Verification items for the finished model (mm, model axes). Face numbers are marked on the shaded views. A direction names the side the tool comes from. Give positions to 0.01 mm unless a question says otherwise; leave off trailing zeros. Loops run counter-clockwise (first coordinate to the right, second up) from the corner with the lowest first, then second, coordinate; pieces in that order, holes last. Notation, with made-up numbers: (35, 16) - (79, 16) arc R27 ccw to (79, 46) - close; hole circle Ø4 at (73.25, -9). An arc over 180 degrees is marked (long way). One line per item, written item: value. Start each with the question number.
1. Mould release check, pull along X, two halves, no side actions. Record for the marked faces 5 and 6: pulls with the +X half, pulls with the -X half, needs draft (parallel to the pull), parting line crosses it, or undercut.
2. Sectioned sample at C-C (z = 2.4). Count the separate pieces of the cut face and the enclosed holes in it, plus the area to 3 significant figures.
3. Access from +Z, -Z, +X, -X, +Y, -Y to the whole of each face (thin tool, end or side, straight path). Record for the marked faces 1, 2, 3 and 4.
4. Sectioned sample at D-D (x = 10). Record the cut outline in (y, z), plus the area to 3 significant figures.
5. Sectioned sample at B-B (y = 0). Record the cut outline in (x, z).
6. Gauge pin test, flat ends, axial feed: pin 1 (1.2 mm diameter, centred on y = 21, z = 2.5, fed in from +X); pin 2 (1.2 mm diameter, centred on x = 0.5, z = 2, fed in from -Y); pin 3 (3 mm diameter, centred on y = -2.5, z = 2, fed in from -X). Record the tip position at first contact, or that the pin passes through.
7. Sectioned sample at A-A (x = -1). Record the cut outline in (y, z).
8. Scan lines: L1, parallel to Y at x = 3, z = 2.85; L2, parallel to X at y = 21, z = 2.4; L3, parallel to X at y = 10, z = 3.75. Record each from-to range of solid material in increasing order. Write a range as [from, to].
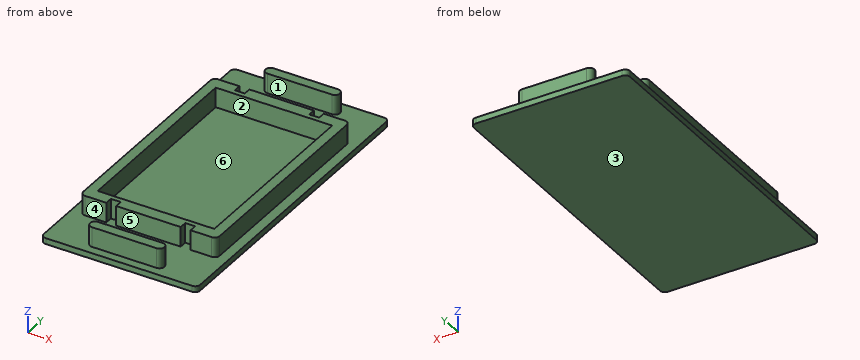
from build123d import *

# Parameters (mm, degrees)
F0_W     = 31.5
F0_H     = 63.5
F0_W_2   = 23.5
F0_H_2   = 39
F0_W_3   = 15
F0_H_3   = 2
F0_W_4   = 2
F0_H_4   = 1.5
F1_DEPTH = 1.2
F2_DEPTH = 4
F3_R     = 0.99999


# Not quite as in the source:
# - a fillet or chamfer is up to 0.001 mm smaller than in the source, because OpenCascade refuses the exact size


with BuildPart() as f1:
    # F0 (on Top) → F1 (new body)
    with BuildSketch(Plane.XY):
        Rectangle(F0_W, F0_H)
        Polygon((13.75, -22), (13.75, -30), (7.5, -30), (-7.5, -30), (-13.75, -30), (-13.75, -22), (-13.75, 22), (-13.75, 30), (-7.5, 30), (7.5, 30), (13.75, 30), (13.75, 22), align=None, mode=Mode.SUBTRACT)
        Rectangle(F0_W_2, F0_H_2)
        Polygon((-7.5, -28), (7.5, -28), (11.75, -28), (11.75, -22), (8.5, -22), (6.5, -22), (-6.5, -22), (-8.5, -22), (-11.75, -22), (-11.75, -28), align=None)
        Polygon((8.5, 22), (11.75, 22), (11.75, 28), (7.5, 28), (-7.5, 28), (-11.75, 28), (-11.75, 22), (-8.5, 22), (-6.5, 22), (6.5, 22), align=None)
        Polygon((-13.75, 22), (-13.75, -22), (-11.75, -22), (-11.75, -19.5), (-11.75, 19.5), (-11.75, 22), align=None)
        Polygon((11.75, -22), (13.75, -22), (13.75, 22), (11.75, 22), (11.75, 19.5), (11.75, -19.5), align=None)
        Polygon((8.5, -22), (11.75, -22), (11.75, -19.5), (-11.75, -19.5), (-11.75, -22), (-8.5, -22), (-8.5, -20.5), (-6.5, -20.5), (-6.5, -22), (6.5, -22), (6.5, -20.5), (8.5, -20.5), align=None)
        Polygon((11.75, 19.5), (11.75, 22), (8.5, 22), (8.5, 20.5), (6.5, 20.5), (6.5, 22), (-6.5, 22), (-6.5, 20.5), (-8.5, 20.5), (-8.5, 22), (-11.75, 22), (-11.75, 19.5), align=None)
        with Locations((0, -29)):
            Rectangle(F0_W_3, F0_H_3)
        with Locations((0, 29)):
            Rectangle(F0_W_3, F0_H_3)
        Polygon((7.5, -30), (13.75, -30), (13.75, -22), (11.75, -22), (11.75, -28), (7.5, -28), align=None)
        Polygon((-13.75, -30), (-7.5, -30), (-7.5, -28), (-11.75, -28), (-11.75, -22), (-13.75, -22), align=None)
        Polygon((11.75, 22), (13.75, 22), (13.75, 30), (7.5, 30), (7.5, 28), (11.75, 28), align=None)
        Polygon((-13.75, 30), (-13.75, 22), (-11.75, 22), (-11.75, 28), (-7.5, 28), (-7.5, 30), align=None)
        with Locations((-7.5, 21.25)):
            Rectangle(F0_W_4, F0_H_4)
        with Locations((7.5, 21.25)):
            Rectangle(F0_W_4, F0_H_4)
        with Locations((-7.5, -21.25)):
            Rectangle(F0_W_4, F0_H_4)
        with Locations((7.5, -21.25)):
            Rectangle(F0_W_4, F0_H_4)
    extrude(amount=-F1_DEPTH)

    # F0 (on Top) → F2 (join)
    with BuildSketch(Plane.XY):
        Polygon((-13.75, 22), (-13.75, -22), (-11.75, -22), (-11.75, -19.5), (-11.75, 19.5), (-11.75, 22), align=None)
        Polygon((11.75, 19.5), (11.75, 22), (8.5, 22), (8.5, 20.5), (6.5, 20.5), (6.5, 22), (-6.5, 22), (-6.5, 20.5), (-8.5, 20.5), (-8.5, 22), (-11.75, 22), (-11.75, 19.5), align=None)
        Polygon((11.75, -22), (13.75, -22), (13.75, 22), (11.75, 22), (11.75, 19.5), (11.75, -19.5), align=None)
        Polygon((8.5, -22), (11.75, -22), (11.75, -19.5), (-11.75, -19.5), (-11.75, -22), (-8.5, -22), (-8.5, -20.5), (-6.5, -20.5), (-6.5, -22), (6.5, -22), (6.5, -20.5), (8.5, -20.5), align=None)
        with Locations((0, 29)):
            Rectangle(F0_W_3, F0_H_3)
        with Locations((0, -29)):
            Rectangle(F0_W_3, F0_H_3)
    extrude(amount=F2_DEPTH)

    # F3 (radius 1 in the source; OpenCascade refuses exactly that, so slightly less here)
    f3_edges = [f1.edges().sort_by_distance(p)[0] for p in [
        (-13.75, 22, 2),
        (13.75, 22, 2),
        (13.75, -22, 2),
        (-13.75, -22, 2),
        (-15.75, -31.75, -0.6),
        (15.75, -31.75, -0.6),
        (-15.75, 31.75, -0.6),
        (15.75, 31.75, -0.6),
        (-7.5, -30, 2),
        (7.5, -30, 2),
        (7.5, -28, 2),
        (-7.5, -28, 2),
        (-7.5, 28, 2),
        (7.5, 28, 2),
        (7.5, 30, 2),
        (-7.5, 30, 2),
    ]]
    fillet(f3_edges, radius=F3_R)


solid = f1.part
Results are:
1. face 5: needs draft
1. face 6: undercut
2. separate pieces: 3
2. enclosed holes: 1
2. area: 339 mm^2
3. face 1: +Z, +X, -X
3. face 2: +Z
3. face 3: -Z, +X, -X, +Y, -Y
3. face 4: +Z, +X, -X, -Y
4. outline: (-31.75, -1.2) - (31.75, -1.2) - (31.75, 0) - (22, 0) - (22, 4) - (19.5, 4) - (19.5, 0) - (-19.5, 0) - (-19.5, 4) - (-22, 4) - (-22, 0) - (-31.75, 0) - close
4. area: 96.2 mm^2
5. outline: (-15.75, -1.2) - (15.75, -1.2) - (15.75, 0) - (13.75, 0) - (13.75, 4) - (11.75, 4) - (11.75, 0) - (-11.75, 0) - (-11.75, 4) - (-13.75, 4) - (-13.75, 0) - (-15.75, 0) - close
6. pin 1: stops at x = 13.75
6. pin 2: stops at y = -30
6. pin 3: stops at x = -13.75
7. outline: (-31.75, -1.2) - (31.75, -1.2) - (31.75, 0) - (30, 0) - (30, 4) - (28, 4) - (28, 0) - (22, 0) - (22, 4) - (19.5, 4) - (19.5, 0) - (-19.5, 0) - (-19.5, 4) - (-22, 4) - (-22, 0) - (-28, 0) - (-28, 4) - (-30, 4) - (-30, 0) - (-31.75, 0) - close
8. L1: y = [-30, -28], [-22, -19.5], [19.5, 22], [28, 30]
8. L2: x = [-13.75, -8.5], [-6.5, 6.5], [8.5, 13.75]
8. L3: x = [-13.75, -11.75], [11.75, 13.75]
